Could you check a few things on this model? Use its own coordinates, in mm. A direction names the side the tool comes from. Coordinates: 2 decimals unless noted, no trailing zeros. Write each loop counter-clockwise with the first axis right and the second up, starting at its lowest first coordinate (ties: lowest second). Pieces come first, ordered by that corner, then holes.
Item 1: If I drill on probe 1 along X at (y, z) = (6.25, 40.5); probe 2 along Z at (x, y) = (221.75, 4.75); probe 3 along X at (y, z) = (10, 40.5), over which ranges is the centre line in solid material (lowest first)?
Item 2: For P1, Ø1.8, axis at x = 221.5, y = 11, coming from the +Z side; P2, Ø1.5, axis at y = 13, z = 51.5, coming from the +X side; P3, Ø3, axis at x = 221, z = 48.5, coming from the -Y side; P4, Ø3.5, axis at x = 221.17, y = 7.5, coming from the -Z side, each with a flat end and sliding along its axis, tell me the tip position at first contact or that it passes through.
Item 3: I want a section at D-D on z = 54.5. Please give me the cut outline in (x, y).
Item 4: I want a section at B-B on z = 40.5. State how many separate pieces and enclosed holes the cut face has, then the cut area to 3 significant figures.
Item 5: Which directions (+Z, -Z, +X, -X, +Y, -Y) give clear straight access to the entire face, cutting with the end or side of a thin tool? Please do faces 5 (the flat face through (221, 12, 50)), 6 (the flat face through (221, 10, 48)).
Item 6: Thinking about a two-plate mould opening in X: for faces 1 (the cylindrical face through (223.267, 7.592, 40.423)), 2 (the flat face through (218.269, 8, 43)), 3 (the flat face through (231.582, 13.336, 45.311)), 4 (the flat face through (239.11, 8.67, 48.41)), which applies, +X half, -X half, draft (parallel to the pull), parting line (faces both ways), or undercut?
Item 7: I want a section at C-C on x = 232.25. Please give me the cut outline in (y, z), then the cut area to 3 significant figures.
Item 8: I want a section at A-A on y = 6. Please give me the cut outline in (x, z).
from build123d import *

# Parameters (mm, degrees)
CYLINDER127_R     = 1.6
CYLINDER127_DEPTH = 40
CYLINDER124_R     = 1.6
CYLINDER124_DEPTH = 40
CYLINDER181_R     = 2.1
CYLINDER181_DEPTH = 19
EXTRUDE067_DEPTH  = 5
EXTRUDE050_DEPTH  = 15
EXTRUDE049_DEPTH  = 21


with BuildPart() as cylinder127:
    # Cylinder127 → Cylinder127 (new body)
    with BuildSketch(Plane(origin=(5.3, 42, 40.5), x_dir=(0, 0, -1), z_dir=(0, -1, 0))):
        Circle(CYLINDER127_R)
    extrude(amount=CYLINDER127_DEPTH)


with BuildPart() as cylinder124:
    # Cylinder124 → Cylinder124 (new body)
    with BuildSketch(Plane(origin=(8.3, 42, 54.5), x_dir=(0, 0, -1), z_dir=(0, -1, 0))):
        Circle(CYLINDER124_R)
    extrude(amount=CYLINDER124_DEPTH)


with BuildPart() as cylinder181:
    # Cylinder181 → Cylinder181 (new body)
    with BuildSketch(Plane(origin=(16.8, 7.5, 32.7), x_dir=(1, 0, 0), z_dir=(0, 0, 1))):
        Circle(CYLINDER181_R)
    extrude(amount=CYLINDER181_DEPTH)


with BuildPart() as cut213:
    # Sketch055 → Extrude067 (new body)
    with BuildSketch(Plane.YZ):
        Polygon((3, 46), (10, 46), (10, 50), (13.646271, 50), (12.6, 35), (3, 35), align=None)
    extrude(amount=EXTRUDE067_DEPTH)


with BuildPart() as cut213_1:
    # Extrude067 placement: moved
    add(cut213.part.moved(Location((14.7, 0, 0))))

    # Cut213: cut Cylinder181
    add(cylinder181.part, mode=Mode.SUBTRACT)


with BuildPart() as extrude050:
    # Sketch040 → Extrude050 (new body)
    with BuildSketch(Plane.XZ):
        Polygon((-8.16038, 62.64716), (-8.16038, 30.419451), (4.410427, 62.64716), align=None)
    extrude(amount=-EXTRUDE050_DEPTH)


with BuildPart() as extrude050_1:
    # Extrude050 placement: moved
    add(extrude050.part.moved(Location((0, 1.5, 0))))


with BuildPart() as cut215:
    # Sketch039 → Extrude049 (new body)
    with BuildSketch(Plane.YZ):
        Polygon((3, 62), (3, 35), (12.616711, 35), (14.5, 62), align=None)
    extrude(amount=EXTRUDE049_DEPTH)


with BuildPart() as cut215_1:
    # Extrude049 placement: moved
    add(cut215.part.moved(Location((-6.3, 0, 0))))

    # Cut212: cut Extrude050
    add(extrude050_1.part, mode=Mode.SUBTRACT)

    # Fusion101: union Cut213
    add(cut213_1.part)

    # Cut214: cut Cylinder124
    add(cylinder124.part, mode=Mode.SUBTRACT)

    # Cut215: cut Cylinder127
    add(cylinder127.part, mode=Mode.SUBTRACT)


with BuildPart() as part_mirroring:
    # Part__Mirroring: instance of Cut215
    add(cut215_1.part.mirror(Plane(origin=(118.984314, 8.749394, 41.218285), x_dir=(0, -1, 0), z_dir=(1, 0, 0))))


solid = part_mirroring.part
Response values:
1. probe 1: x = 218.27 to 219.48, 222.86 to 231.07, 234.27 to 242.2
1. probe 2: z = 35 to 46
1. probe 3: x = 218.27 to 231.07, 234.27 to 242.2
2. P1: stops at z = 50
2. P2: stops at x = 238.2
2. P3: stops at y = 10
2. P4: passes through
3. outline: (223.27, 3) - (228.07, 3) - (228.07, 13.98) - (223.27, 13.98) - close; (231.27, 3) - (236.74, 3) - (236.74, 13.98) - (231.27, 13.98) - close
4. separate pieces: 2
4. enclosed holes: 1
4. area: 193 mm2
5. face 5: +Z, -X, +Y, -Y
5. face 6: +Z, -X, -Y
6. face 1: undercut
6. face 2: -X half
6. face 3: draft
6. face 4: +X half
7. outline: (3, 35) - (12.62, 35) - (12.89, 38.96) - (3, 38.96) - close; (3, 42.04) - (13.11, 42.04) - (14.5, 62) - (3, 62) - close
7. area: 254 mm2
8. outline: (218.27, 35) - (219.7, 35) - (219.7, 46) - (218.27, 46) - close; (222.64, 35) - (244.27, 35) - (244.27, 35.19) - (233.81, 62) - (223.27, 62) - (223.27, 46) - (222.64, 46) - close; hole circle Ø3.2 at (229.67, 54.5); hole circle Ø3.2 at (232.67, 40.5)
